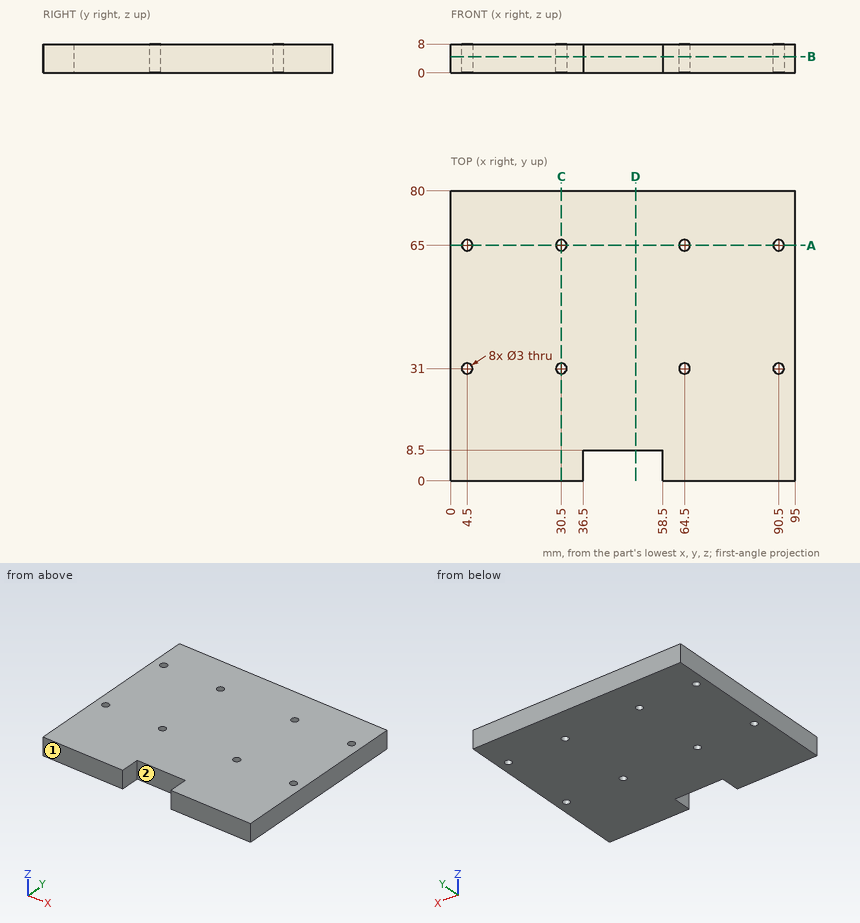
Design review of the part shown in the three views and the two pictorial views. Dimensions are in mm from the part's minimum x, y and z. Give positions to 0.01 mm unless a question says otherwise; leave off trailing zeros. Loops run counter-clockwise (first coordinate to the right, second up) from the corner with the lowest first, then second, coordinate; pieces in that order, holes last. Notation, with made-up numbers: (-2, -9) - (30, -9) arc R14 cw to (30, 3) - close; hole circle Ø3 at (34.25, 0.5). An arc over 180 degrees is marked (long way). Write item = value, one per line.
1) Clearance check with flat-ended pins moving along their axes: pin 1 Ø1.8 at (x, y) = (4.5, 65) entering from +Z; pin 2 Ø4 at (x, y) = (4.5, 31) entering from +Z; pin 3 Ø4 at (x, z) = (53, 3.5) entering from -Y. State where each tip first meets the part, or that it passes through.
Result sheet:
pin_1 = through
pin_2 = 8
pin_3 = 8.5
2) To check wall thickness, follow line 1 (X direction, y = 65, z = 1.75); line 2 (Y direction, x = 90.5, z = 2.75); line 3 (Y direction, x = 91.5, z = 0.5). State the ranges of each line that lie inside material, in increasing order.
Result sheet:
line_1 = 0 to 3, 6 to 29, 32 to 63, 66 to 89, 92 to 95
line_2 = 0 to 29.5, 32.5 to 63.5, 66.5 to 80
line_3 = 0 to 29.88, 32.12 to 63.88, 66.12 to 80
3) Take a section at C-C on x = 30.5. State the section outline as (y, z) points.
Result sheet:
outline = (0, 0) - (29.5, 0) - (29.5, 8) - (0, 8) - close; (32.5, 0) - (63.5, 0) - (63.5, 8) - (32.5, 8) - close; (66.5, 0) - (80, 0) - (80, 8) - (66.5, 8) - close
4) Draft analysis for pull direction X (two halves, no side actions). For the marked faces 1 and 2, state which applies: +X half, -X half, draft (parallel to the pull), parting line (faces both ways), or undercut.
Result sheet:
face_1 = draft
face_2 = undercut
5) Take a section at D-D on x = 51. State the section outline as (y, z) points, and give its area (3 significant figures).
Result sheet:
outline = (8.5, 0) - (80, 0) - (80, 8) - (8.5, 8) - close
area = 572 mm2
6) Take a section at A-A on y = 65. State the section outline as (x, z) points.
Result sheet:
outline = (0, 0) - (3, 0) - (3, 8) - (0, 8) - close; (6, 0) - (29, 0) - (29, 8) - (6, 8) - close; (32, 0) - (63, 0) - (63, 8) - (32, 8) - close; (66, 0) - (89, 0) - (89, 8) - (66, 8) - close; (92, 0) - (95, 0) - (95, 8) - (92, 8) - close
7) Take a section at B-B on z = 4.5. Count the separate pieces of the cut face and the enclosed holes in it, and give its area (3 significant figures).
Result sheet:
separate_pieces = 1
enclosed_holes = 8
area = 7,360 mm2
